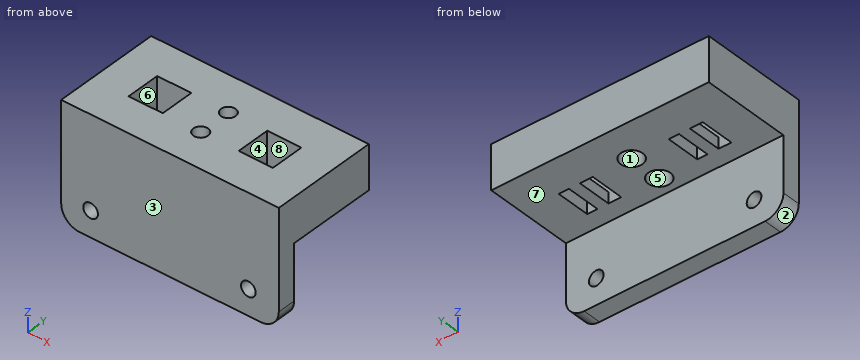
```python
from build123d import *

# Parameters (mm, degrees)
BOX004_W               = 3
BOX004_H               = 10
BOX004_DEPTH           = 3
CYLINDER005_R          = 2
CYLINDER005_DEPTH      = 3
CYLINDER001_R          = 3
CYLINDER001_DEPTH      = 10
CYLINDER006_R          = 2
CYLINDER006_DEPTH      = 3
CYLINDER004_R          = 3
CYLINDER004_DEPTH      = 10
BOX_W                  = 9.3
BOX_H                  = 9.3
BOX_DEPTH              = 12
BOX005_W               = 9.3
BOX005_H               = 9.3
BOX005_DEPTH           = 12
BOX003_W               = 59.3
BOX003_H               = 29.3
BOX003_DEPTH           = 12
CYLINDER002_R          = 2
CYLINDER002_DEPTH      = 10
CYLINDER002_ROLL_ANGLE = 90
CYLINDER003_R          = 2
CYLINDER003_DEPTH      = 10
CYLINDER003_ROLL_ANGLE = 90
BOX006_W               = 59.3
BOX006_H               = 5
BOX006_DEPTH           = 20
FILLET_R               = 5
BOX001_W               = 3
BOX001_H               = 10
BOX001_DEPTH           = 3


with BuildPart() as cube004:
    # Box004 → Box004 (new body)
    with BuildSketch(Plane(origin=(33.5, 0, 0), x_dir=(1, 0, 0), z_dir=(0, 0, 1))):
        with Locations((1.5, 5)):
            Rectangle(BOX004_W, BOX004_H)
    extrude(amount=BOX004_DEPTH)


with BuildPart() as cylinder005:
    # Cylinder005 → Cylinder005 (new body)
    with BuildSketch(Plane(origin=(19.65, 9, 5), x_dir=(1, 0, 0), z_dir=(0, 0, 1))):
        Circle(CYLINDER005_R)
    extrude(amount=CYLINDER005_DEPTH)


with BuildPart() as cylinder001:
    # Cylinder001 → Cylinder001 (new body)
    with BuildSketch(Plane(origin=(19.65, 9, -5), x_dir=(1, 0, 0), z_dir=(0, 0, 1))):
        Circle(CYLINDER001_R)
    extrude(amount=CYLINDER001_DEPTH)


with BuildPart() as cylinder006:
    # Cylinder006 → Cylinder006 (new body)
    with BuildSketch(Plane(origin=(19.65, 0, 5), x_dir=(1, 0, 0), z_dir=(0, 0, 1))):
        Circle(CYLINDER006_R)
    extrude(amount=CYLINDER006_DEPTH)


with BuildPart() as fusion003:
    # Cylinder004 → Cylinder004 (new body)
    with BuildSketch(Plane(origin=(19.65, 0, -5), x_dir=(1, 0, 0), z_dir=(0, 0, 1))):
        Circle(CYLINDER004_R)
    extrude(amount=CYLINDER004_DEPTH)

    # Fusion003: union Cylinder005, Cylinder001, Cylinder006
    add(cylinder005.part)
    add(cylinder001.part)
    add(cylinder006.part)


with BuildPart() as fusion003_1:
    # Fusion003 placement: moved
    add(fusion003.part.moved(Location((0, 0, 4))))


with BuildPart() as cube:
    # Box → Box (new body)
    with BuildSketch(Plane(origin=(30, 0, 0), x_dir=(1, 0, 0), z_dir=(0, 0, 1))):
        with Locations((4.65, 4.65)):
            Rectangle(BOX_W, BOX_H)
    extrude(amount=BOX_DEPTH)


with BuildPart() as fusion:
    # Box005 → Box005 (new body)
    with BuildSketch(Plane.XY):
        with Locations((4.65, 4.65)):
            Rectangle(BOX005_W, BOX005_H)
    extrude(amount=BOX005_DEPTH)

    # Fusion: union Cube
    add(cube.part)


with BuildPart() as cut001:
    # Box003 → Box003 (new body)
    with BuildSketch(Plane(origin=(-10, -10, 0), x_dir=(1, 0, 0), z_dir=(0, 0, 1))):
        with Locations((29.65, 14.65)):
            Rectangle(BOX003_W, BOX003_H)
    extrude(amount=BOX003_DEPTH)

    # Cut: cut Fusion
    add(fusion.part, mode=Mode.SUBTRACT)

    # Cut001: cut Fusion003
    add(fusion003_1.part, mode=Mode.SUBTRACT)


with BuildPart() as cylinder002:
    # Cylinder002 → Cylinder002 (new body)
    with BuildSketch(Plane.XY):
        Circle(CYLINDER002_R)
    extrude(amount=CYLINDER002_DEPTH)


with BuildPart() as cylinder002_1:
    # Cylinder002 roll: moved
    add(cylinder002.part.rotate(Axis((0, 0, 0), (1, 0, 0)), CYLINDER002_ROLL_ANGLE))


with BuildPart() as cylinder002_2:
    # Cylinder002 placement: moved
    add(cylinder002_1.part.moved(Location((-2, 0, -13))))


with BuildPart() as fusion002:
    # Cylinder003 → Cylinder003 (new body)
    with BuildSketch(Plane.XY):
        Circle(CYLINDER003_R)
    extrude(amount=CYLINDER003_DEPTH)


with BuildPart() as fusion002_1:
    # Cylinder003 roll: moved
    add(fusion002.part.rotate(Axis((0, 0, 0), (1, 0, 0)), CYLINDER003_ROLL_ANGLE))


with BuildPart() as fusion002_2:
    # Cylinder003 placement: moved
    add(fusion002_1.part.moved(Location((41, 0, -13))))

    # Fusion002: union Cylinder002
    add(cylinder002_2.part)


with BuildPart() as cut002:
    # Box006 → Box006 (new body)
    with BuildSketch(Plane(origin=(-10, -10, -20), x_dir=(1, 0, 0), z_dir=(0, 0, 1))):
        with Locations((29.65, 2.5)):
            Rectangle(BOX006_W, BOX006_H)
    extrude(amount=BOX006_DEPTH)

    # Fillet
    fillet_edges = [cut002.edges().sort_by_distance(p)[0] for p in [
        (-10, -7.5, -20),
        (49.3, -7.5, -20),
    ]]
    fillet(fillet_edges, radius=FILLET_R)

    # Cut002: cut Fusion002
    add(fusion002_2.part, mode=Mode.SUBTRACT)


with BuildPart() as fusion004:
    # Box001 → Box001 (new body)
    with BuildSketch(Plane(origin=(3.5, 0, 0), x_dir=(1, 0, 0), z_dir=(0, 0, 1))):
        with Locations((1.5, 5)):
            Rectangle(BOX001_W, BOX001_H)
    extrude(amount=BOX001_DEPTH)

    # Fusion004: union Cube004, Cut001, Cut002
    add(cube004.part)
    add(cut001.part)
    add(cut002.part)


solid = fusion004.part
```
Work out the finished part from the listing and answer in its coordinate system (mm). Face numbers are marked on the shaded views. A direction names the side the tool comes from. Give positions to 0.01 mm unless a question says otherwise; leave off trailing zeros. Loops run counter-clockwise (first coordinate to the right, second up) from the corner with the lowest first, then second, coordinate; pieces in that order, holes last. Notation, with made-up numbers: (40, -6) -> (93, -6) arc R17 ccw to (93, 6) -> close; hole circle Ø7 at (-19.75, 32.5). An arc over 180 degrees is marked (long way). Write item = value, one per line. Start each with the question number.
(1) Given pin 1 Ø6.5 at (x, y) = (20.5, 9) entering from -Z; pin 2 Ø5 at (x, z) = (41, -13) entering from +Y; pin 3 Ø3.5 at (x, y) = (34.5, 5) entering from +Z, each flat-ended and moving along its own axis, determine where each tip first touches the part or whether it passes through.
(2) Find section C-C on z = 4. Give the vertices of the cut face in (x, y).
(3) Which of the six approach directions +Z, -Z, +X, -X, +Y, -Y give full straight-line access (tool end or side, diameter ignored) to the marked faces 5, 6, 7 and 8?
(4) The mould has two halves that part along Y. Classify the marked faces 1, 2, 3 and 4: +Y half, -Y half, draft (parallel to the pull), parting line (faces both ways), or undercut.
(5) Find section A-A on x = -2. Give the vertices of the cut face in (y, z), and give its area (3 significant figures).
(6) Find section B-B on y = 4.75. Give the vertices of the cut face in (x, z), and give its area (3 significant figures).
(7) Find the intervals of material crossed by probe 1 along X at (y, z) = (9, 3.25); probe 2 along X at (y, z) = (-8.4, -13); probe 3 along Y at (x, z) = (19.65, 7), in increasing order. Write a range as from..to.
(8) Find section D-D on z = -13. Give the vertices of the cut face in (x, y), and give its area (4 significant figures).
From the geometry:
q1.pin_1 = 0
q1.pin_2 = -5
q1.pin_3 = 3
q2.outline = (-10, -10) -> (49.3, -10) -> (49.3, 19.3) -> (-10, 19.3) -> close; hole (0, 0) -> (9.3, 0) -> (9.3, 9.3) -> (0, 9.3) -> close; hole circle Ø6 at (19.65, 0); hole circle Ø6 at (19.65, 9); hole (30, 0) -> (39.3, 0) -> (39.3, 9.3) -> (30, 9.3) -> close
q3.face_5 = -Z
q3.face_6 = +Z, -Z
q3.face_7 = -Z, +X, -X, +Y
q3.face_8 = +Z
q4.face_1 = undercut
q4.face_2 = draft
q4.face_3 = -Y half
q4.face_4 = undercut
q5.outline = (-10, -20) -> (-5, -20) -> (-5, -15) -> (-10, -15) -> close; (-10, -11) -> (-5, -11) -> (-5, 0) -> (19.3, 0) -> (19.3, 12) -> (-10, 12) -> close
q5.area = 432 mm^2
q6.outline = (-10, 0) -> (0, 0) -> (0, 12) -> (-10, 12) -> close; (3.5, 0) -> (6.5, 0) -> (6.5, 3) -> (3.5, 3) -> close; (9.3, 0) -> (30, 0) -> (30, 12) -> (9.3, 12) -> close; (33.5, 0) -> (36.5, 0) -> (36.5, 3) -> (33.5, 3) -> close; (39.3, 0) -> (49.3, 0) -> (49.3, 12) -> (39.3, 12) -> close
q6.area = 506 mm^2
q7.probe_1 = -10..0, 9.3..16.65, 22.65..30, 39.3..49.3
q7.probe_2 = -10..-4, 0..39, 43..49.3
q7.probe_3 = -10..-3, 3..6, 12..19.3
q8.outline = (-10, -10) -> (-4, -10) -> (-4, -5) -> (-10, -5) -> close; (0, -10) -> (39, -10) -> (39, -5) -> (0, -5) -> close; (43, -10) -> (49.3, -10) -> (49.3, -5) -> (43, -5) -> close
q8.area = 256.5 mm^2
